For this review, take the finished solid that the model builds, in its own axes (mm). A direction names the side the tool comes from. Round coordinates to 2 decimals unless told otherwise and drop trailing zeros. Loops run counter-clockwise (first coordinate to the right, second up) from the corner with the lowest first, then second, coordinate; pieces in that order, holes last.
1) Take a section at B-B (x = 5). State the section outline as (y, z) points.
2) Tool access review of faces 4 (the flat face through (34, 4, -13.002)), 5 (the flat face through (34, 6.597, -9)), 6 (the flat face through (54.8, 45, -15)), 7 (the flat face through (69.8, 5, -24)): name each direction out of +Z, -Z, +X, -X, +Y, -Y from which nothing blocks a thin tool from reaching the whole face with its end or side.
3) Insertion check: pin 1 (4 mm diameter, centred on x = 13.5, z = -5.5, fed in from +Y); pin 2 (8 mm diameter, centred on y = 46, z = -13, fed in from +X); pin 3 (6.5 mm diameter, centred on x = 32, y = 3, fed in from -Z). Each pin has a flat end and moves straight along its axis. Give the tip position at first contact, or say it passes through.
4) Wall thickness on L1, parallel to Y at x = 19.5, z = -7.5; L2, parallel to X at y = 52, z = -24; L3, parallel to Y at x = 40, z = -10: over which ranges is each line inside the solid? List them lowest first.
5) Take a section at D-D (x = 37.5). State the section outline as (y, z) points.
6) Take a section at A-A (y = 12.5). State the section outline as (x, z) points.
7) Take a section at C-C (x = 79.55). State the section outline as (y, z) points.
8) Mouldability with a two-part tool opening along Y and no side actions: class faces 1 (the flat face through (34, 26.997, -15)), 2 (the flat face through (53, 57.997, -15)), 3 (the flat face through (70, 22, -33.402)) as pulls with the +Y half, pulls with the -Y half, needs draft (parallel to the pull), parting line crosses it, or undercut.
Autodesk Inventor part; units mm, degrees
ref_plane "YZ Plane" through (0, 0, 0) normal (1, 0, 0) x (0, 1, 0)
ref_plane "XZ Plane" through (0, 0, 0) normal (0, 1, 0) x (-1, 0, 0)
ref_plane "XY Plane" through (0, 0, 0) normal (0, 0, 1) x (1, 0, 0)
sketch "Sketch2" plane through (0, 0, 0) normal (1, 0, 0) x (0, 1, 0)
  line L0 (26.9971, -5.0019) -> (6.5971, -5.0019)
  line L1 (6.5971, -5.0019) -> (6.5971, -25.4019)
  line L2 (6.5971, -25.4019) -> (26.9971, -25.4019)
  line L3 (26.9971, -25.4019) -> (26.9971, -5.0019)
  line L4 (30.9971, -2.0019) -> (0.5971, -2.0019)
  line L5 (30.9971, -28.4019) -> (30.9971, -2.0019)
  line L6 (0.5971, -2.0019) -> (0.5971, -28.4019)
  line L7 (30.9971, -28.4019) -> (0.5971, -28.4019)
  line L8 (6.5971, -13.0019) -> (0.5971, -13.0019)
  line L9 (0.5971, -13.0019) -> (0.5971, -17.4019)
  line L10 (0.5971, -17.4019) -> (6.5971, -17.4019)
  line L11 (6.5971, -17.4019) -> (6.5971, -13.0019)
  point P0 (0, 0)
  point P1 (0.5971, -13.0019)
  dimension "d5" = 20.4
  dimension "d6" = 20.4
  dimension "d8" = 6
  dimension "d22" = 4
  dimension "d23" = 3
  dimension "d24" = 3
  dimension "d27" = 8
  dimension "d28" = 8
extrude "Extrusion1" add sketch "Sketch2" along normal blind 54.8 contours L0 L1 L8 L6 L4 L5 L7 L10 L2 L3
sketch "Sketch4" plane through (0, 0.5971, -28.4019) normal (0, 0, -1) x (-1, 0, 0)
  line L0 (0, 6) -> (0, 26.4)
  line L1 (0, 26.4) -> (-54.8, 26.4)
  line L2 (-54.8, 6) -> (-54.8, 26.4)
  line L3 (0, 6) -> (-54.8, 6)
  line L4 (0, 26.4) -> (-54.8, 26.4)
  line L5 (-54.8, 26.4) -> (-83.55, 26.4)
  line L6 (-83.55, 26.4) -> (-83.55, 16.4)
  line L7 (-83.55, 16.4) -> (-54.8, 16.4)
  line L8 (-54.8, 16.4) -> (-54.8, 26.4)
  line L9 (-43.55, 26.4) -> (-43.55, 16.4) construction
  point P0 (0, -0.5971)
  dimension "d29" = 10
  dimension "d30" = 11.25
  dimension "d31" = 40
  dimension "d32" = 0
extrude "Extrusion3" add sketch "Sketch4" along normal blind 5 and the other way blind 3 contours L2 L7 L6 L5
sketch "Sketch10" plane through (54.8, 26.9971, -33.4019) normal (0, 1, 0) x (1, 0, 0)
  line L0 (28.75, -8) -> (0, -8)
  line L1 (28.75, -8) -> (28.75, 0)
  line L2 (0, 0) -> (28.75, 0)
  line L3 (0, 0) -> (0, -5)
  circle A0 centre (24.75, -4) radius 1.5
  line L4 (0, -8) -> (0, -5)
  point P0 (-54.8, -33.4019)
  dimension "d55" = 3
  dimension "d56" = 4
  dimension "d57" = 4
extrude "Extrusion8" cut sketch "Sketch10" against normal blind 10 contours A0
sketch "Sketch11" plane through (54.8, 0, 0) normal (1, 0, 0) x (0, 0, -1)
  line L0 (25.4019, 26.9971) -> (28.4019, 26.9971)
  line L1 (28.4019, 26.9971) -> (28.4019, 30.9971)
  line L2 (28.4019, 30.9971) -> (2.0019, 30.9971)
  line L3 (2.0019, 30.9971) -> (2.0019, 0.5971)
  line L4 (2.0019, 0.5971) -> (13.0019, 0.5971)
  line L5 (13.0019, 0.5971) -> (13.0019, 6.5971)
  line L6 (13.0019, 6.5971) -> (5.0019, 6.5971)
  line L7 (5.0019, 6.5971) -> (5.0019, 26.9971)
  line L8 (5.0019, 26.9971) -> (25.4019, 26.9971)
  line L9 (28.4019, 16.9971) -> (25.4019, 16.9971)
  line L10 (25.4019, 16.9971) -> (25.4019, 6.5971)
  line L11 (25.4019, 6.5971) -> (17.4019, 6.5971)
  line L12 (17.4019, 6.5971) -> (17.4019, 0.5971)
  line L13 (17.4019, 0.5971) -> (28.4019, 0.5971)
  line L14 (28.4019, 0.5971) -> (28.4019, 16.9971)
  point P0 (0, 0)
extrude "Extrusion9" add sketch "Sketch11" along normal blind 15
fillet "Fillet3" radius 2 6 edges at (62.3, 26.9971, -28.4019) (54.8, 21.9971, -28.4019) (62.3, 16.9971, -28.4019) (69.8, 26.9971, -26.9019) (69.8, 16.9971, -26.9019) (54.8, 21.9971, -33.4019)
sketch "Sketch12" plane through (0, 0.5971, -28.4019) normal (0, 0, -1) x (-1, 0, 0)
  line L0 (0, 0) -> (0, 6)
  line L1 (0, 6) -> (-69.8, 6)
  line L2 (-69.8, 0) -> (-69.8, 6)
  line L3 (0, 0) -> (-69.8, 0)
  circle A0 centre (-64.8, 3) radius 1.1
  circle A1 centre (-40.8, 3) radius 1.1
  circle A2 centre (-5, 3) radius 1.1
  point P0 (0, -0.5971)
  dimension "d64" = 2.2
  dimension "d65" = 5
  dimension "d66" = 3
  dimension "d67" = 2.2
  dimension "d68" = 2.2
  dimension "d69" = 5
  dimension "d70" = 3
  dimension "d71" = 29
  dimension "d72" = 3
extrude "Extrusion10" cut sketch "Sketch12" against normal blind 100 contours A0 | A1 | A2
sketch "Sketch13" plane through (0, 30.9971, -2.0019) normal (0, 1, 0) x (1, 0, 0)
  line L0 (0, 0) -> (69.8, 0)
  line L1 (0, 26.4) -> (69.8, 26.4)
  line L2 (54.8, 0) -> (50.8, 0)
  line L3 (50.8, 0) -> (50.8, 26.4)
  line L4 (50.8, 26.4) -> (54.8, 26.4)
  line L5 (54.8, 26.4) -> (54.8, 0)
  line L6 (4, 0) -> (0, 0)
  line L7 (0, 0) -> (0, 26.4)
  line L8 (0, 26.4) -> (4, 26.4)
  line L9 (4, 26.4) -> (4, 0)
  line L10 (0, 26.4) -> (0, 0)
  point P0 (0, -2.0019)
  point P1 (4, 0)
  point P2 (50.8, 0)
  dimension "d75" = 4
  dimension "d76" = 4
  dimension "d77" = 46.8
extrude "Extrusion11" add sketch "Sketch13" along normal blind 27 contours L7 L1 L9 L0 | L3 L1 L5 L0
sketch "Sketch14" plane through (54.8, 30.9971, -2.0019) normal (1, 0, 0) x (0, 0, -1)
  circle A0 centre (5.2, 11) radius 1.3
  line L0 (26.4, 0) -> (0, 0)
  circle A1 centre (5.2, 23) radius 1.3
  line L1 (0, 0) -> (0, 27)
  circle A2 centre (21.2, 23) radius 1.3
  circle A3 centre (21.2, 11) radius 1.3
  line L2 (26.4, 0) -> (26.4, 27)
  point P0 (-2.0019, -30.9971)
  dimension "d80" = 2.6
  dimension "d81" = 11
  dimension "d82" = 2.6
  dimension "d83" = 23
  dimension "d86" = 2.6
  dimension "d87" = 2.6
  dimension "d88" = 11
  dimension "d89" = 23
  dimension "d95" = 16
  dimension "d96" = 16
  dimension "d97" = 5.2
  dimension "d98" = 5.2
extrude "Extrusion12" cut sketch "Sketch14" against normal blind 100
fillet "Fillet4" radius 2 1 edges at (54.8, 30.9971, -15.2019)
equation "\"d98\" = d97"
properties part number "Motor_mount"
Response:
1. outline: (0.6, -28.4) - (2.5, -28.4) - (2.5, -17.4) - (0.6, -17.4) - close; (0.6, -13) - (2.5, -13) - (2.5, -2) - (0.6, -2) - close; (4.7, -28.4) - (31, -28.4) - (31, -2) - (4.7, -2) - (4.7, -13) - (6.6, -13) - (6.6, -5) - (27, -5) - (27, -25.4) - (6.6, -25.4) - (6.6, -17.4) - (4.7, -17.4) - close
2. face 4: +X, -X, -Y
2. face 5: +X, -X
2. face 6: +Z, -Z, +X, +Y
2. face 7: +Z, -Z, +X, -Y
3. pin 1: stops at y = 31
3. pin 2: stops at x = 54.8
3. pin 3: stops at z = -28.4
4. L1: y = 0.6 to 6.6, 27 to 31
4. L2: x = 0 to 4, 50.8 to 54.8
4. L3: y = 0.6 to 2.84, 4.35 to 6.6, 27 to 31
5. outline: (0.6, -28.4) - (31, -28.4) - (31, -2) - (0.6, -2) - (0.6, -13) - (6.6, -13) - (6.6, -5) - (27, -5) - (27, -25.4) - (6.6, -25.4) - (6.6, -17.4) - (0.6, -17.4) - close
6. outline: (0, -28.4) - (69.8, -28.4) - (69.8, -25.4) - (0, -25.4) - close; (0, -5) - (69.8, -5) - (69.8, -2) - (0, -2) - close
7. outline: (17, -33.4) - (27, -33.4) - (27, -30.9) - (17, -30.9) - close; (17, -27.9) - (27, -27.9) - (27, -25.4) - (17, -25.4) - close
8. face 1: undercut
8. face 2: pulls with the +Y half
8. face 3: needs draft
